Build history of the part. All positions in model axes, mm. Coordinates: 2 decimals unless noted, no trailing zeros. Order: outer loops, then holes, each group sorted by start corner. A loop starts at its lowest first (then second) coordinate and runs counter-clockwise, first axis right, second up. Notation, with made-up numbers: (50.25, 65) - (100.25, 65) arc R16 cw to (100.25, 72) - close; hole circle Ø8 at (-17, 3.25). An arc over 180 degrees is marked (long way). Return JSON: item names as keys, results as strings.
Autodesk Inventor part; units mm, degrees
ref_plane "YZ Plane" through (0, 0, 0) normal (1, 0, 0) x (0, 1, 0)
ref_plane "XZ Plane" through (0, 0, 0) normal (0, 1, 0) x (-1, 0, 0)
ref_plane "XY Plane" through (0, 0, 0) normal (0, 0, 1) x (1, 0, 0)
sketch "Boceto1" plane through (0, 0, 0) normal (0, 1, 0) x (-1, 0, 0)
  line L0 (4.925, -3.9) -> (4.925, -4.2)
  line L1 (4.925, -4.2) -> (2.025, -4.2)
  line L2 (2.025, -4.2) -> (2.025, -3.9)
  line L3 (2.025, -3.9) -> (4.925, -3.9)
  line L4 (-4.925, -3.3) -> (-2.025, -3.3)
  line L5 (-2.025, -3.3) -> (-2.025, -3.6)
  line L6 (-2.025, -3.6) -> (-4.925, -3.6)
  line L7 (-4.925, -3.6) -> (-4.925, -3.3)
  line L8 (3, 2.4695) -> (3, 2.7695)
  line L9 (3, 2.7695) -> (5.7, 2.7695)
  line L10 (5.7, 2.7695) -> (5.7, 2.4695)
  line L11 (5.7, 2.4695) -> (3, 2.4695)
  line L12 (3, 3.0695) -> (3, 3.3695)
  line L13 (3, 3.3695) -> (5.4, 3.3695)
  line L14 (5.4, 3.3695) -> (5.4, 3.0695)
  line L15 (5.4, 3.0695) -> (3, 3.0695)
  line L16 (2.025, -5.4) -> (3.825, -5.4)
  line L17 (3.825, -5.4) -> (3.825, -5.7)
  line L18 (3.825, -5.7) -> (2.025, -5.7)
  line L19 (2.025, -5.7) -> (2.025, -5.4)
  line L20 (-3.825, -5.7) -> (-3.825, -5.4)
  line L21 (-3.825, -5.4) -> (-2.025, -5.4)
  line L22 (-2.025, -5.4) -> (-2.025, -5.7)
  line L23 (-2.025, -5.7) -> (-3.825, -5.7)
  line L24 (-3.825, -6.3) -> (-3.825, -6)
  line L25 (-3.825, -6) -> (-2.025, -6)
  line L26 (-2.025, -6) -> (-2.025, -6.3)
  line L27 (-2.025, -6.3) -> (-3.825, -6.3)
  line L28 (2.025, -6.3) -> (2.025, -6)
  line L29 (2.025, -6) -> (3.825, -6)
  line L30 (3.825, -6) -> (3.825, -6.3)
  line L31 (3.825, -6.3) -> (2.025, -6.3)
  line L32 (-3, 3.3695) -> (-3, 3.0695)
  line L33 (-3, 3.0695) -> (-5.4, 3.0695)
  line L34 (-5.4, 3.0695) -> (-5.4, 3.3695)
  line L35 (-5.4, 3.3695) -> (-3, 3.3695)
  line L36 (-3, 2.7695) -> (-3, 2.4695)
  line L37 (-3, 2.4695) -> (-5.7, 2.4695)
  line L38 (-5.7, 2.4695) -> (-5.7, 2.7695)
  line L39 (-5.7, 2.7695) -> (-3, 2.7695)
  line L40 (-4.925, -4.2) -> (-4.925, -3.9)
  line L41 (-4.925, -3.9) -> (-2.025, -3.9)
  line L42 (-2.025, -3.9) -> (-2.025, -4.2)
  line L43 (-2.025, -4.2) -> (-4.925, -4.2)
  line L44 (4.925, -3.6) -> (2.025, -3.6)
  line L45 (2.025, -3.6) -> (2.025, -3.3)
  line L46 (2.025, -3.3) -> (4.925, -3.3)
  line L47 (4.925, -3.3) -> (4.925, -3.6)
  line L48 (0.15, -6.5) -> (-0.15, -6.5)
  line L49 (-1.2, -6.5) -> (-1.5, -6.5)
  line L50 (1.5, -6.5) -> (1.2, -6.5)
  line L51 (-6.725, -2.7) -> (-6.725, 1.7)
  line L52 (-6.725, 1.7) -> (-4.325, 1.7)
  line L53 (-4.325, 1.7) -> (-4.325, -2.7)
  line L54 (-4.325, -2.7) -> (-6.725, -2.7)
  line L55 (4.3, -2.7) -> (4.3, 1.7)
  line L56 (4.3, 1.7) -> (6.7, 1.7)
  line L57 (6.7, 1.7) -> (6.7, -2.7)
  line L58 (6.7, -2.7) -> (4.3, -2.7)
  circle A0 centre (-4.734, 4.334) radius 0.1
  circle A1 centre (4.734, 4.334) radius 0.1
  circle A2 centre (-4.734, -5.334) radius 0.1
  circle A3 centre (4.734, -5.334) radius 0.1
  circle A4 centre (-3.8, 0.894) radius 0.1
  circle A5 centre (-3.8, -1.894) radius 0.1
  circle A6 centre (3.8, 0.894) radius 0.1
  circle A7 centre (3.8, -1.894) radius 0.1
  line L59 (2.55, -1.4) -> (-2.55, -1.4)
  line L60 (1.5, -1.4) -> (1.5, -6.5)
  line L61 (1.2, -6.5) -> (1.2, -1.4)
  line L62 (0.15, -1.4) -> (0.15, -6.5)
  line L63 (-0.15, -6.5) -> (-0.15, -1.4)
  line L64 (-1.5, -6.5) -> (-1.5, -1.4)
  line L65 (-1.2, -1.4) -> (-1.2, -6.5)
  line L66 (2.55, -1.4) -> (2.55, 6.6532)
  line L67 (-2.55, -1.4) -> (-2.55, 6.6532)
  line L68 (-7.5, -0.5) -> (-7.5, -0.4)
  line L69 (7.5, -0.5) -> (7.5, -0.4)
  line L70 (-7.5, -0.5) -> (-7.5, -0.6)
  line L71 (7.4993, -0.5) -> (7.4993, -0.6)
  arc A8 (-7.5, -0.6) -> (7.4993, -0.6) centre (-0.0003, -0.6) ccw
  arc A9 (7.4993, -0.5) -> (2.55, 6.6532) centre (0, -0.4) ccw
  arc A10 (-2.55, 6.6532) -> (-7.5, -0.4) centre (0, -0.4) ccw
  line L72 (-4.734, -5.184) -> (-5.4457, -5.184)
  line L73 (-4.734, -5.234) -> (-4.734, -5.334)
  point P0 (2.352, 6.909)
  dimension "d43" = 0.2
  dimension "d13" = 0.1
  dimension "d14" = 0.1
  dimension "d15" = 0.1
  dimension "d39" = 0.2
  dimension "d40" = 0.2
  dimension "d41" = 0.2
  dimension "d42" = 0.2
  dimension "d44" = 0.2
  dimension "d45" = 0.2
  dimension "d46" = 0.2
extrude "Extrusión1" add sketch "Boceto1" along normal blind 0.3 contours L62 L59 L61 L50 L60 L66 A9 L69 L71 A8 L70 L68 A10 L67 L64 L49 L65 L63 L48
sketch "Boceto2" plane through (0, 0.3, 0) normal (0, 1, 0) x (1, 0, 0)
  line L0 (-1.2, 6.5) -> (-1.2, 1.4)
  line L1 (-1.5, 1.4) -> (-1.5, 6.5)
  line L2 (-0.15, 1.4) -> (-0.15, 6.5)
  line L3 (0.15, 6.5) -> (0.15, 1.4)
  line L4 (1.2, 1.4) -> (1.2, 6.5)
  line L5 (1.5, 6.5) -> (1.5, 1.4)
  line L6 (1.2, 6.5) -> (1.5, 6.5)
  line L7 (-0.15, 6.5) -> (0.15, 6.5)
  line L8 (-1.5, 6.5) -> (-1.2, 6.5)
  line L9 (-1.5, 6.5) -> (-1.2, 6.5)
  line L10 (-1.2, 6.5) -> (-1.2, 1.4)
  line L11 (-1.2, 1.4) -> (-1.5, 1.4)
  line L12 (-1.5, 1.4) -> (-1.5, 6.5)
  line L13 (-0.15, 6.5) -> (0.15, 6.5)
  line L14 (0.15, 6.5) -> (0.15, 1.4)
  line L15 (0.15, 1.4) -> (-0.15, 1.4)
  line L16 (-0.15, 1.4) -> (-0.15, 6.5)
  line L17 (1.2, 6.5) -> (1.5, 6.5)
  line L18 (1.5, 6.5) -> (1.5, 1.4)
  line L19 (1.5, 1.4) -> (1.2, 1.4)
  line L20 (1.2, 1.4) -> (1.2, 6.5)
  point P0 (0, 0)
extrude "Extrusión2" add sketch "Boceto2" along normal mid plane 0.6
sketch "Boceto3" plane through (-2.4, 0, -1.4) normal (0, 0, 1) x (1, 0, 0)
  line L0 (0, 0) -> (4.8, 0)
  line L1 (0, 0.3) -> (4.8, 0.3)
  line L2 (0, 0.3) -> (4.8, 0.3)
  line L3 (9.9, 0.3) -> (-5.1, 0.3)
  line L4 (4.8, 0) -> (0, 0)
  line L5 (9.9, 0) -> (-5.1, 0)
  line L6 (-0.3, 0.15) -> (-0.15, 0)
  line L7 (-0.3, 0.15) -> (-0.15, 0.3)
  line L8 (5.1, 0.15) -> (4.95, 0.3)
  line L9 (5.1, 0.15) -> (4.95, 0)
  line L10 (-0.15, 0.3) -> (4.95, 0.3)
  line L11 (4.95, 0) -> (-0.15, 0)
  point P0 (2.4, 0)
  point P1 (0.048, 0)
  point P2 (4.752, 0)
extrude "Extrusión3" cut sketch "Boceto3" along normal blind 10
sketch "Boceto4" plane through (0, 0.3, 0) normal (0, 1, 0) x (1, 0, 0)
  circle A0 centre (-0.675, 7) radius 0.15
  line L0 (4.325, -1.7) -> (4.325, 2.7)
  circle A1 centre (0.675, 7) radius 0.15
  line L1 (-6.7, -1.7) -> (-6.7, 2.7)
  line L2 (-6.7, 2.7) -> (-4.3, 2.7)
  line L3 (-4.3, 2.7) -> (-4.3, -1.7)
  line L4 (-4.3, -1.7) -> (-6.7, -1.7)
  line L5 (4.325, 2.7) -> (6.725, 2.7)
  line L6 (6.725, 2.7) -> (6.725, -1.7)
  line L7 (-3.825, 5.8) -> (-2.025, 5.8)
  line L8 (-2.025, 5.5) -> (-3.825, 5.5)
  line L9 (2.025, 5.8) -> (3.825, 5.8)
  line L10 (3.825, 5.5) -> (2.025, 5.5)
  line L11 (4.325, 2.7) -> (6.725, 2.7)
  line L12 (2.025, 6.3) -> (3.825, 6.3)
  circle A2 centre (-0.675, 7) radius 0.1
  circle A3 centre (0.675, 7) radius 0.1
  point P0 (0, 0)
  dimension "d47" = 0.3
  dimension "d48" = 0.2
  dimension "d49" = 0.2
extrude "Extrusión4" cut sketch "Boceto4" against normal blind 10 contours A2 | A3
sketch "Boceto8" plane through (0, 0.3, 0) normal (0, 1, 0) x (1, 0, 0)
  circle A0 centre (-3.8, -0.894) radius 0.1
  line L0 (0, 0) -> (0, -2.4412)
  circle A1 centre (3.8, -0.894) radius 0.1
  circle A2 centre (3.6, 4.906) radius 0.15
  circle A3 centre (-3.6, 4.906) radius 0.15
  dimension "d33" = 0.3
  dimension "d34" = 0.3
extrude "Extrusión6" cut sketch "Boceto8" against normal blind 10 contours A2 | A3
sketch "Boceto9" plane through (0, 0, 0) normal (0, -1, 0) x (1, 0, 0)
  line L0 (-2.85, 3.6695) -> (-4.09, 3.6695)
  line L1 (-4.09, 5.5295) -> (-4.09, 3.6695)
  line L2 (-2.85, 3.6695) -> (-2.85, 5.5295)
  line L3 (-4.09, 5.5295) -> (-2.85, 5.5295)
  line L4 (-3, 3.3695) -> (-5.4, 3.3695)
  line L5 (-2.55, 6.6532) -> (-2.55, -1.4)
  point P0 (0, 0)
extrude "Extrusión7" cut sketch "Boceto9" against normal blind 10
sketch "Boceto11" plane through (0, 0, 0) normal (0, -1, 0) x (1, 0, 0)
  line L0 (-2.85, 5.5295) -> (-4.09, 5.5295)
  line L1 (-2.85, 5.5295) -> (-3.15, 5.5295)
  line L2 (-3.15, 5.5295) -> (-3.15, 5.5795)
  line L3 (-4.09, 5.5295) -> (-3.79, 5.5295)
  line L4 (-3.79, 5.5295) -> (-3.79, 5.5795)
  line L5 (-3.79, 5.5795) -> (-3.15, 5.5795)
  line L6 (-4.09, 5.5295) -> (-4.09, 3.6695)
  line L7 (-4.09, 3.6695) -> (-4.09, 5.5295)
  line L8 (-2.85, 3.6695) -> (-3.15, 3.6695)
  line L9 (-3.15, 3.6695) -> (-3.15, 3.6195)
  line L10 (-4.09, 3.6695) -> (-3.79, 3.6695)
  line L11 (-3.79, 3.6695) -> (-3.79, 3.6195)
  line L12 (-3.79, 3.6195) -> (-3.15, 3.6195)
  line L13 (-2.85, 5.5295) -> (-2.85, 3.6695)
  point P0 (0, 0)
  dimension "d50" = 0.3
  dimension "d51" = 0.05
  dimension "d52" = 0.3
  dimension "d53" = 0.05
extrude "Extrusión8" cut sketch "Boceto11" against normal blind 10
properties part number "LBase"
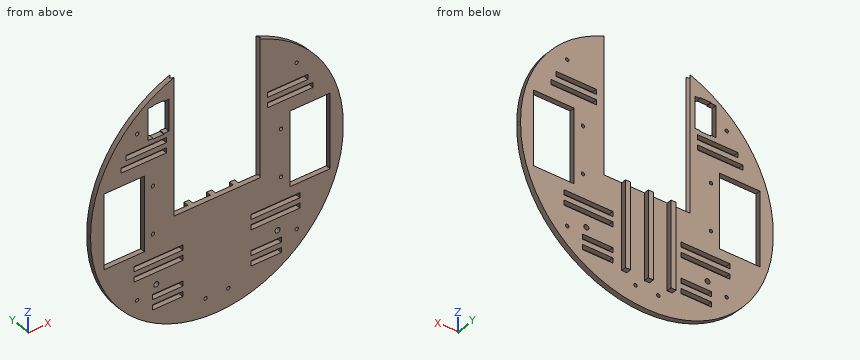
1. Drop a flat-ended pin along its axis: pin 1 (1 mm diameter, centred on x = 5.5, z = -5.5, fed in from +Y). Give the stop position or say it passes through.
Check values:
{"pin 1": "y = 0.3"}
2. Cut at A-A on y = 0.4. Give the cut face in (x, z), plus the area to 3 significant figures.
Check values:
{"outline": "(-1.5, -6.5) - (-1.2, -6.5) - (-1.2, -1.4) - (-1.5, -1.4) - close; (-0.15, -6.5) - (0.15, -6.5) - (0.15, -1.4) - (-0.15, -1.4) - close; (1.2, -6.5) - (1.5, -6.5) - (1.5, -1.4) - (1.2, -1.4) - close", "area": "4.59 mm²"}
3. Cut at B-B on z = -2.25. Give the cut face in (x, y) (3 decimals).
Check values:
{"outline": "(-7.316, 0) - (-6.7, 0) - (-6.7, 0.3) - (-7.316, 0.3) - close; (-4.3, 0) - (4.325, 0) - (4.325, 0.3) - (1.5, 0.3) - (1.5, 0.6) - (1.2, 0.6) - (1.2, 0.3) - (0.15, 0.3) - (0.15, 0.6) - (-0.15, 0.6) - (-0.15, 0.3) - (-1.2, 0.3) - (-1.2, 0.6) - (-1.5, 0.6) - (-1.5, 0.3) - (-4.3, 0.3) - close; (6.725, 0) - (7.316, 0) - (7.316, 0.3) - (6.725, 0.3) - close"}
4. Probe L1, parallel to X at y = 0.45, z = -4; L2, parallel to X at y = 0.1, z = -5.5 (3 decimals); L3, parallel to Z at x = -2.5, y = 0.05. List the from-to ranges inside material, lowest first.
Check values:
{"L1": "-1.5 to -1.2, -0.15 to 0.15, 1.2 to 1.5", "L2": "-5.677 to -3.825, -2.025 to 2.025, 3.825 to 5.678", "L3": "-7.67 to -6.3, -6 to -5.7, -5.4 to -4.2, -3.9 to -3.6, -3.3 to -1.4"}
5. Cut at D-D on z = 0.5. Give the cut face in (x, y) (3 decimals).
Check values:
{"outline": "(-7.446, 0) - (-6.7, 0) - (-6.7, 0.3) - (-7.446, 0.3) - close; (-4.3, 0) - (-2.55, 0) - (-2.7, 0.15) - (-2.55, 0.3) - (-4.3, 0.3) - close; (2.55, 0) - (4.325, 0) - (4.325, 0.3) - (2.55, 0.3) - (2.7, 0.15) - close; (6.725, 0) - (7.446, 0) - (7.446, 0.3) - (6.725, 0.3) - close"}
6. Cut at C-C on x = 6.25. Give the cut face in (y, z), plus the area to 3 significant figures.
Check values:
{"outline": "(0, -4.75) - (0.3, -4.75) - (0.3, -2.7) - (0, -2.7) - close; (0, 1.7) - (0.3, 1.7) - (0.3, 3.75) - (0, 3.75) - close", "area": "1.23 mm²"}
